Input: part model. Units: mm. Frame: model coordinates. A direction names the side the tool comes from. Round coordinates to 2 decimals unless told otherwise and drop trailing zeros. Order: outer loops, then holes, each group sorted by start corner. A loop starts at its lowest first (then second) coordinate and runs counter-clockwise, first axis right, second up. Notation, with made-up numbers: (58.5, 88) -> (99.5, 88) arc R19 cw to (99.5, 99) -> close; hole circle Ø1 at (-6.5, 3). An arc over 180 degrees is marked (long way). Use a Markdown table: item, result.
from build123d import *

# Parameters (mm, degrees)
ESBO_O1_W                = 10
ESBO_O1_H                = 4
ESBO_O1_W_2              = 35
ESBO_O1_H_2              = 32
ESBO_O1_R                = 2.6
RESSALTO_EXTRUS_O1_DEPTH = 6


with BuildPart() as part:
    # Esboço1 → Ressalto-extrusão1 (new body)
    with BuildSketch(Plane.XY):
        with Locations((-12.5, -18)):
            Rectangle(ESBO_O1_W, ESBO_O1_H)
        Rectangle(ESBO_O1_W_2, ESBO_O1_H_2)
        with Locations((-12.5, 0)):
            Circle(ESBO_O1_R, mode=Mode.SUBTRACT)
        with Locations((12.5, 0)):
            Circle(ESBO_O1_R, mode=Mode.SUBTRACT)
        with Locations((12.5, -18)):
            Rectangle(ESBO_O1_W, ESBO_O1_H)
        with Locations((12.5, 18)):
            Rectangle(ESBO_O1_W, ESBO_O1_H)
        with Locations((-12.5, 18)):
            Rectangle(ESBO_O1_W, ESBO_O1_H)
    extrude(amount=RESSALTO_EXTRUS_O1_DEPTH)


solid = part.part
1) Ray query, probe 1 along Y at (x, z) = (-12.5, 4.5); probe 2 along Y at (x, z) = (-14, 3.5); probe 3 along Y at (x, z) = (-5.5, 4.4). Return the intervals inside material, ascending.
Answer key:
| item | result |
|---|---|
| probe 1 | y = -20 to -2.6, 2.6 to 20 |
| probe 2 | y = -20 to -2.12, 2.12 to 20 |
| probe 3 | y = -16 to 16 |
2) Cut plane D-D on y = -16.5. Return loops of the section in (x, z).
Answer key:
| item | result |
|---|---|
| outline | (-17.5, 0) -> (-7.5, 0) -> (-7.5, 6) -> (-17.5, 6) -> close; (7.5, 0) -> (17.5, 0) -> (17.5, 6) -> (7.5, 6) -> close |
3) Cut plane A-A on x = 12.5. Return loops of the section in (y, z), and give its area (3 significant figures).
Answer key:
| item | result |
|---|---|
| outline | (-20, 0) -> (-2.6, 0) -> (-2.6, 6) -> (-20, 6) -> close; (2.6, 0) -> (20, 0) -> (20, 6) -> (2.6, 6) -> close |
| area | 209 mm^2 |
4) Contact query for flat-ended pins moving along their axis: P1, Ø2, axis at x = -8.5, y = -13.5, coming from the -Z side; P2, Ø1.8, axis at x = 0.5, z = 4, coming from the +Y side; P3, Ø3, axis at x = 2.5, z = 2, coming from the -Y side. Output: stop coordinate, or through.
Answer key:
| item | result |
|---|---|
| P1 | stops at z = 0 |
| P2 | stops at y = 16 |
| P3 | stops at y = -16 |
5) Cut plane B-B on z = 4.4. Return loops of the section in (x, y), and give its area (3 significant figures).
Answer key:
| item | result |
|---|---|
| outline | (-17.5, -20) -> (-7.5, -20) -> (-7.5, -16) -> (7.5, -16) -> (7.5, -20) -> (17.5, -20) -> (17.5, 20) -> (7.5, 20) -> (7.5, 16) -> (-7.5, 16) -> (-7.5, 20) -> (-17.5, 20) -> close; hole circle Ø5.2 at (-12.5, 0); hole circle Ø5.2 at (12.5, 0) |
| area | 1,240 mm^2 |
6) Set-up query: faces 4 (the face through (0, 0, 0)), 5 (the face through (-7.5, -18, 3)), 6 (the face through (-7.5, 18, 3)). Return all of +Z, -Z, +X, -X, +Y, -Y with unobstructed straight access to the full face (end or side cutting, diameter ignored); none if empty.
Answer key:
| item | result |
|---|---|
| face 4 | -Z, +X, -X, +Y, -Y |
| face 5 | +Z, -Z, -Y |
| face 6 | +Z, -Z, +Y |
7) Draft query along X for faces 1 (the face through (14.98, 0.78, 2.96)), 2 (the face through (12, -20, 3)), 3 (the face through (17.5, 0, 3)). Return one class per face: released by +X, released by -X, zero draft, split by the parting line, or undercut.
Answer key:
| item | result |
|---|---|
| face 1 | undercut |
| face 2 | zero draft |
| face 3 | released by +X |
8) Cut plane C-C on y = 0. Return loops of the section in (x, z), and give its area (3 significant figures).
Answer key:
| item | result |
|---|---|
| outline | (-17.5, 0) -> (-15.1, 0) -> (-15.1, 6) -> (-17.5, 6) -> close; (-9.9, 0) -> (9.9, 0) -> (9.9, 6) -> (-9.9, 6) -> close; (15.1, 0) -> (17.5, 0) -> (17.5, 6) -> (15.1, 6) -> close |
| area | 148 mm^2 |
